Geometry check sheet. Reference: drawing and pictorial views, mm from the part's lowest x, y, z. A direction names the side the tool comes from. Coordinates: 2 decimals unless noted, no trailing zeros. Write each loop counter-clockwise with the first axis right and the second up, starting at its lowest first coordinate (ties: lowest second). Pieces come first, ordered by that corner, then holes.
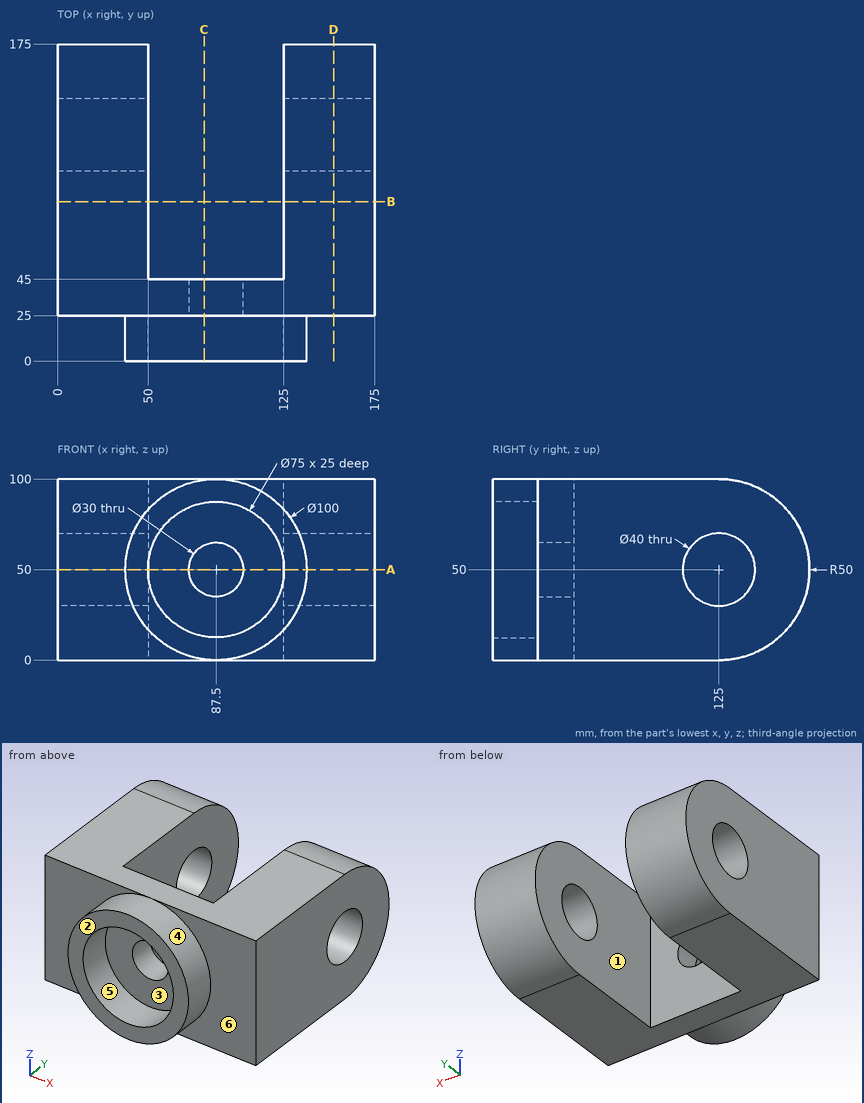
1. Sectioned sample at D-D, the plane x = 152.5. Record the boundary of the cut face in (y, z).
2. Draft check along X on the marked faces 4, 5 and 6. Enter one of: pulls with the +X half, pulls with the -X half, needs draft (parallel to the pull), parting line crosses it, or undercut.
3. Sectioned sample at B-B, the plane y = 88. Record the boundary of the cut face in (x, z).
4. Material ranges on L1, parallel to X at y = 90.5, z = 61; L2, parallel to Y at x = 23, z = 50; L3, parallel to X at y = 14, z = 50, recorded low to high.
5. Tool access check on the marked faces 1, 2 and 3. Record the directions out of +Z, -Z, +X, -X, +Y, -Y that give a thin tool (end or side, any length) a straight path to the whole face; none if there is none.
6. Gauge pin test, flat ends, axial feed: P1, Ø8, axis at x = 29.5, z = 65, coming from the +Y side (3 decimals); P2, Ø3, axis at x = 119, z = 44.5, coming from the +Y side; P3, Ø18, axis at x = 87.5, z = 50, coming from the +Y side. Record the tip position at first contact, or that the pin passes through.
7. Sectioned sample at C-C, the plane x = 81. Record the boundary of the cut face in (y, z).
8. Sectioned sample at A-A, the plane z = 50. Record the boundary of the cut face in (x, y), and give its area (3 significant figures).
Outcome:
1. outline: (25, 0) - (125, 0) arc R50 ccw to (125, 100) - (25, 100) - close; hole circle Ø40 at (125, 50)
2. face 4: parting line crosses it
2. face 5: undercut
2. face 6: needs draft
3. outline: (0, 0) - (50, 0) - (50, 100) - (0, 100) - close; (125, 0) - (175, 0) - (175, 100) - (125, 100) - close
4. L1: x = 0 to 50, 125 to 175
4. L2: y = 25 to 105, 145 to 175
4. L3: x = 37.5 to 50, 125 to 137.5
5. face 1: +Z, -Z, +Y
5. face 2: +Z, -Z, +X, -X, -Y
5. face 3: -Y
6. P1: stops at y = 173.775
6. P2: stops at y = 45
6. P3: passes through
7. outline: (0, 0.42) - (25, 0.42) - (25, 0) - (45, 0) - (45, 36.48) - (25, 36.48) - (25, 13.07) - (0, 13.07) - close; (0, 86.93) - (25, 86.93) - (25, 63.52) - (45, 63.52) - (45, 100) - (25, 100) - (25, 99.58) - (0, 99.58) - close
8. outline: (0, 25) - (37.5, 25) - (37.5, 0) - (50, 0) - (50, 25) - (72.5, 25) - (72.5, 45) - (50, 45) - (50, 105) - (0, 105) - close; (0, 145) - (50, 145) - (50, 175) - (0, 175) - close; (102.5, 25) - (125, 25) - (125, 0) - (137.5, 0) - (137.5, 25) - (175, 25) - (175, 105) - (125, 105) - (125, 45) - (102.5, 45) - close; (125, 145) - (175, 145) - (175, 175) - (125, 175) - close
8. area: 12,500 mm2
